```python
from build123d import *

# Parameters (mm, degrees)
BOSS_EXTRUDE1_DEPTH = 152
SKETCH2_W           = 20
SKETCH2_H           = 10.5
CUT_EXTRUDE1_DEPTH  = 11
CUT_EXTRUDE2_DEPTH  = 5
SKETCH7_R           = 2.6
CUT_EXTRUDE3_DEPTH  = 6


with BuildPart() as part:
    # Sketch1 → Boss-Extrude1 (new body)
    with BuildSketch(Plane.XY):
        Polygon((-33.5, 0), (-33.5, 10), (33.5, 10), (33.5, 0), (7.5, 0), (7.5, 2.5), (-7.5, 2.5), (-7.5, 0), align=None)
    extrude(amount=BOSS_EXTRUDE1_DEPTH)

    # Sketch2 → Cut-Extrude1 (cut, through all)
    with BuildSketch(Plane(origin=(0, 10, 0), x_dir=(1, 0, 0), z_dir=(0, 1, 0))):
        with Locations((0, -5.25)):
            Rectangle(SKETCH2_W, SKETCH2_H)
    extrude(amount=-CUT_EXTRUDE1_DEPTH, mode=Mode.SUBTRACT)

    # Sketch6 → Cut-Extrude2 (cut)
    with BuildSketch(Plane(origin=(0, 10, 0), x_dir=(1, 0, 0), z_dir=(0, 1, 0))):
        with BuildLine():
            Line((-26.44, 0), (-30.56, 0))
            ThreePointArc((-30.56, 0), (-28.5, -8.50079992), (-26.44, 0))
        make_face()
    cut_extrude2 = extrude(amount=-CUT_EXTRUDE2_DEPTH, mode=Mode.SUBTRACT)

    # Sketch7 → Cut-Extrude3 (cut, through all)
    with BuildSketch(Plane(origin=(0, 5, 0), x_dir=(1, 0, 0), z_dir=(0, 1, 0))):
        with Locations((-28.5, -4.00079992)):
            Circle(SKETCH7_R)
    cut_extrude3 = extrude(amount=-CUT_EXTRUDE3_DEPTH, mode=Mode.SUBTRACT)

    # Mirror1: Cut-Extrude2, Cut-Extrude3 across plane
    add(cut_extrude2.mirror(Plane(origin=(0, 0, 0), x_dir=(0, 0, 1), z_dir=(1, 0, 0))), mode=Mode.SUBTRACT)
    add(cut_extrude3.mirror(Plane(origin=(0, 0, 0), x_dir=(0, 0, 1), z_dir=(1, 0, 0))), mode=Mode.SUBTRACT)


solid = part.part
```
The model under review builds one solid part; all positions refer to its coordinate system, in mm. A direction names the side the tool comes from. Round coordinates to 2 decimals unless told otherwise and drop trailing zeros. Order: outer loops, then holes, each group sorted by start corner. A loop starts at its lowest first (then second) coordinate and runs counter-clockwise, first axis right, second up.
Item 1: Add section D-D, the plane x = -5. State the section outline as (y, z) points.
Working result:
outline: (2.5, 10.5) - (10, 10.5) - (10, 152) - (2.5, 152) - close
Item 2: Add section C-C, the plane x = 28. State the section outline as (y, z) points, and give its area (3 significant figures).
Working result:
outline: (0, 0) - (5, 0) - (5, 1.45) - (0, 1.45) - close; (0, 6.55) - (5, 6.55) - (5, 8.47) - (10, 8.47) - (10, 152) - (0, 152) - close
area: 1,450 mm2
Item 3: For pin 1 (8 mm diameter, centred on x = 1, z = 92.5, fed in from -Y), flat-tipped, find the tip position at first contact; note if it passes through.
Working result:
pin 1: stops at y = 2.5
Item 4: Add section A-A, the plane x = -28.5. State the section outline as (y, z) points, and give its area (3 significant figures).
Working result:
outline: (0, 0) - (5, 0) - (5, 1.4) - (0, 1.4) - close; (0, 6.6) - (5, 6.6) - (5, 8.5) - (10, 8.5) - (10, 152) - (0, 152) - close
area: 1,450 mm2
Item 5: Draft analysis for pull direction X (two halves, no side actions). For faces 1 (the flat face through (-22, 5, 0)), 2 (the flat face through (7.5, 1, 80)), 3 (the flat face through (33.5, 5, 75)), state which applies: released by +X, released by -X, zero draft, split by the parting line, or undercut.
Working result:
face 1: zero draft
face 2: undercut
face 3: released by +X
Item 6: To check wall thickness, follow probe 1 along Z at (x, y) = (28.5, 3.95); probe 2 along X at (y, z) = (0.5, 51.5); probe 3 along Y at (x, z) = (-1.5, 95). State the ranges of each line that lie inside material, in increasing order.
Working result:
probe 1: z = 0 to 1.4, 6.6 to 152
probe 2: x = -33.5 to -7.5, 7.5 to 33.5
probe 3: y = 2.5 to 10
Item 7: Machinability: for faces 4 (the flat face through (-10, 5, 5)), 5 (the flat face through (0, 10, 75)), 6 (the flat face through (-7.5, 1, 80)), 7 (the cylindrical face through (-31.1, 2.5, 3.9)), 8 (the cylindrical face through (-28.668, 7.535, 8.498)), which of the approach directions +Z, -Z, +X, -X, +Y, -Y give a long, thin tool a straight path to every point of the face, cutting with its end or side? Answer none if there is none.
Working result:
face 4: -Z, +Y, -Y
face 5: +Z, -Z, +X, -X, +Y
face 6: +Z, -Z, -Y
face 7: +Y, -Y
face 8: +Y
Item 8: Add section B-B, the plane z = 48. State the section outline as (x, y) points, and give its area (4 significant figures).
Working result:
outline: (-33.5, 0) - (-7.5, 0) - (-7.5, 2.5) - (7.5, 2.5) - (7.5, 0) - (33.5, 0) - (33.5, 10) - (-33.5, 10) - close
area: 632.5 mm2
